Verification items for the finished model (mm, model axes). Coordinates: 2 decimals unless noted, no trailing zeros. Write each loop counter-clockwise with the first axis right and the second up, starting at its lowest first coordinate (ties: lowest second). Pieces come first, ordered by that corner, then holes. Notation, with made-up numbers: (57.5, 83) -> (95.5, 83) arc R22 cw to (95.5, 116) -> close; hole circle Ø1 at (-24, 32.25). An arc over 180 degrees is marked (long way). Answer in a Markdown table with one row per item.
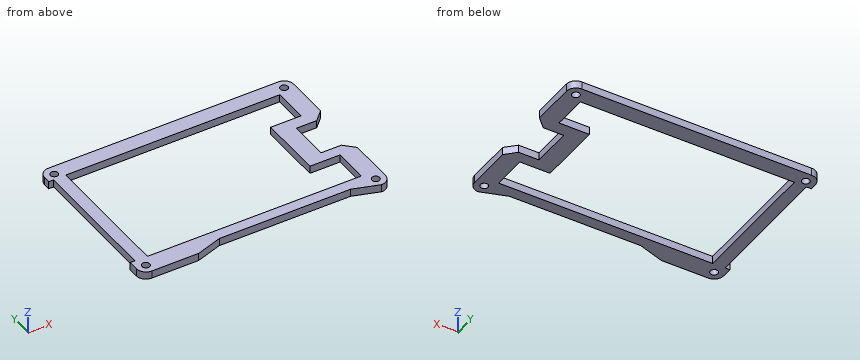
```python
from build123d import *

# Parameters (mm, degrees)
BOSS_EXTRUDE1_DEPTH = 3.048
SKETCH2_R           = 1.355900406
CUT_EXTRUDE1_DEPTH  = 4.048
SKETCH3_R           = 1.524
CUT_EXTRUDE2_DEPTH  = 4.048
CUT_EXTRUDE3_DEPTH  = 4.048
BOSS_EXTRUDE2_DEPTH = 3.048
SKETCH5_W           = 73.1256
SKETCH5_H           = 52.8987
SKETCH5_W_2         = 9.017
SKETCH5_H_2         = 13.74935
CUT_EXTRUDE4_DEPTH  = 4.048
SKETCH6_W           = 3.048
SKETCH6_H           = 13.74935
CUT_EXTRUDE5_DEPTH  = 4.048


with BuildPart() as part:
    # Sketch1 → Boss-Extrude1 (new body)
    with BuildSketch(Plane.XY):
        with BuildLine():
            Line((-309.8086, 128.8851), (-305.87795, 128.8851))
            Line((-305.87795, 128.8851), (-301.9473, 132.81575))
            Line((-301.9473, 132.81575), (-301.9473, 150.9704))
            ThreePointArc((-301.9473, 150.9704), (-303.063223164, 153.664476836), (-305.7573, 154.7804))
            Line((-305.7573, 154.7804), (-397.247125, 154.7804))
            ThreePointArc((-397.247125, 154.7804), (-399.946077222, 153.659592612), (-401.0571, 150.956597849))
            Line((-401.0571, 150.956597849), (-401.0571, 148.341))
            Line((-401.0571, 148.341), (-399.1521, 148.341))
            Line((-399.1521, 148.341), (-399.1521, 95.6449))
            Line((-399.1521, 95.6449), (-401.0571, 95.6449))
            Line((-401.0571, 95.6449), (-401.0571, 91.659304166))
            ThreePointArc((-401.0571, 91.659304166), (-399.951018769, 88.947400452), (-397.2472, 87.8217))
            Line((-397.2472, 87.8217), (-378.5565, 87.8217))
            Line((-378.5565, 87.8217), (-368.3165, 91.1883))
            Line((-368.3165, 91.1883), (-315.9973, 91.1883))
            Line((-315.9973, 91.1883), (-305.7573, 87.8217))
            ThreePointArc((-305.7573, 87.8217), (-303.063223164, 88.937623164), (-301.9473, 91.6317))
            Line((-301.9473, 91.6317), (-301.9473, 111.74645))
            Line((-301.9473, 111.74645), (-305.87795, 115.6771))
            Line((-305.87795, 115.6771), (-309.8086, 115.6771))
            Line((-309.8086, 115.6771), (-314.0123, 115.6771))
            Line((-314.0123, 115.6771), (-314.0123, 128.8851))
            Line((-314.0123, 128.8851), (-309.8086, 128.8851))
        make_face()
        Polygon((-395.3675, 92.9525), (-395.3675, 149.2432), (-309.8086, 149.2432), (-309.8086, 132.81575), (-318.2033, 132.81575), (-318.2033, 111.74645), (-309.8086, 111.74645), (-309.8086, 92.9525), align=None, mode=Mode.SUBTRACT)
    extrude(amount=BOSS_EXTRUDE1_DEPTH)

    # Sketch2 → Cut-Extrude1 (cut, through all)
    with BuildSketch(Plane(origin=(0, 0, 0), x_dir=(-1, 0, 0), z_dir=(0, 0, -1))):
        with Locations((305.7573, 150.9704)):
            Circle(SKETCH2_R)
        with Locations((397.247125, 150.9704)):
            Circle(SKETCH2_R)
        with Locations((397.2472, 91.6317)):
            Circle(SKETCH2_R)
        with Locations((305.7573, 91.6317)):
            Circle(SKETCH2_R)
    extrude(amount=-CUT_EXTRUDE1_DEPTH, mode=Mode.SUBTRACT)

    # Sketch3 → Cut-Extrude2 (cut, through all)
    with BuildSketch(Plane(origin=(0, 0, 0), x_dir=(-1, 0, 0), z_dir=(0, 0, -1))):
        with Locations((305.7573, 150.9704)):
            Circle(SKETCH3_R)
        with Locations((397.247125, 150.9704)):
            Circle(SKETCH3_R)
        with Locations((397.2472, 91.6317)):
            Circle(SKETCH3_R)
        with Locations((305.7573, 91.6317)):
            Circle(SKETCH3_R)
    extrude(amount=-CUT_EXTRUDE2_DEPTH, mode=Mode.SUBTRACT)

    # Sketch4 → Cut-Extrude3 (cut, through all)
    with BuildSketch(Plane.XY.offset(3.048)):
        Polygon((-301.9473, 133.57775), (-305.87795, 129.6471), (-314.0123, 129.6471), (-314.0123, 113.6451), (-305.87795, 113.6451), (-301.9473, 109.71445), align=None)
    extrude(amount=-CUT_EXTRUDE3_DEPTH, mode=Mode.SUBTRACT)

    # Sketch4<4> → Boss-Extrude2 (add)
    with BuildSketch(Plane.XY.offset(3.048)):
        Polygon((-318.2033, 111.74645), (-318.2033, 132.81575), (-309.8086, 132.81575), (-309.8086, 149.2432), (-395.3675, 149.2432), (-395.3675, 92.9525), (-309.8086, 92.9525), (-309.8086, 111.74645), align=None)
    extrude(amount=-BOSS_EXTRUDE2_DEPTH)

    # Sketch5 → Cut-Extrude4 (cut, through all)
    with BuildSketch(Plane.XY.offset(3.048)):
        with Locations((-357.6871, 121.98105)):
            Rectangle(SKETCH5_W, SKETCH5_H)
        with Locations((-316.6158, 141.555725)):
            Rectangle(SKETCH5_W_2, SKETCH5_H_2)
        with Locations((-316.6158, 102.406375)):
            Rectangle(SKETCH5_W_2, SKETCH5_H_2)
    extrude(amount=-CUT_EXTRUDE4_DEPTH, mode=Mode.SUBTRACT)

    # Sketch6 → Cut-Extrude5 (cut, through all)
    with BuildSketch(Plane.XY.offset(3.048)):
        with Locations((-310.5833, 141.555725)):
            Rectangle(SKETCH6_W, SKETCH6_H)
        with Locations((-310.5833, 102.406375)):
            Rectangle(SKETCH6_W, SKETCH6_H)
    extrude(amount=-CUT_EXTRUDE5_DEPTH, mode=Mode.SUBTRACT)


solid = part.part
```
1. Material ranges on probe 1 along Y at (x, z) = (-319, 0.8); probe 2 along Y at (x, z) = (-325.5, 1.05); probe 3 along X at (y, z) = (117.5, 1.8), recorded low to high. Write a range as from..to.
Findings below:
| item | result |
|---|---|
| probe 1 | y = 91.19..95.53, 109.28..134.68, 148.43..154.78 |
| probe 2 | y = 91.19..95.53, 148.43..154.78 |
| probe 3 | x = -399.15..-394.25, -321.12..-314.01 |
2. Sectioned sample at D-D, the plane x = -315. Record the cut outline in (y, z), and give its area (3 significant figures).
Findings below:
| item | result |
|---|---|
| outline | (90.86, 0) -> (95.53, 0) -> (95.53, 3.05) -> (90.86, 3.05) -> close; (109.28, 0) -> (134.68, 0) -> (134.68, 3.05) -> (109.28, 3.05) -> close; (148.43, 0) -> (154.78, 0) -> (154.78, 3.05) -> (148.43, 3.05) -> close |
| area | 111 mm² |
3. Sectioned sample at B-B, the plane x = -387. Record the cut outline in (y, z).
Findings below:
| item | result |
|---|---|
| outline | (87.82, 0) -> (95.53, 0) -> (95.53, 3.05) -> (87.82, 3.05) -> close; (148.43, 0) -> (154.78, 0) -> (154.78, 3.05) -> (148.43, 3.05) -> close |
4. Sectioned sample at A-A, the plane y = 123. Record the cut outline in (x, z), and give its area (3 significant figures).
Findings below:
| item | result |
|---|---|
| outline | (-399.15, 0) -> (-394.25, 0) -> (-394.25, 3.05) -> (-399.15, 3.05) -> close; (-321.12, 0) -> (-314.01, 0) -> (-314.01, 3.05) -> (-321.12, 3.05) -> close |
| area | 36.6 mm² |
5. Sectioned sample at C-C, the plane z = 1.35. Count the separate pieces of the cut face and the enclosed holes in it, and give its area (3 significant figures).
Findings below:
| item | result |
|---|---|
| separate pieces | 1 |
| enclosed holes | 5 |
| area | 1,880 mm² |
6. Go/stop test with flat-tipped pins: pin 1 (4 mm diameter, centred on x = -305.76, y = 150.97, fed in from -Z); pin 2 (0.9 mm diameter, centred on x = -369, z = 1.5, fed in from -Y); pin 3 (1 mm diameter, centred on x = -400, z = 1, fed in from -Y); pin 4 (0.9 mm diameter, centred on y = 123, z = 1.5, fed in from -X). Record where each tip stops, or that it passes through.
Findings below:
| item | result |
|---|---|
| pin 1 | stops at z = 0 |
| pin 2 | stops at y = 90.82 |
| pin 3 | stops at y = 88.56 |
| pin 4 | stops at x = -399.15 |
